Verification items for the finished model (mm, model axes). Face numbers are marked on the shaded views. Round coordinates to 2 decimals unless told otherwise and drop trailing zeros. Write each loop counter-clockwise with the first axis right and the second up, starting at its lowest first coordinate (ties: lowest second). Pieces come first, ordered by that corner, then holes. Notation, with made-up numbers: M -28.5,40 L 10.5,40 A25 cw 10.5,55 Z; hole C 0,83 d4. An arc over 180 degrees is marked long. Use a Markdown table: item, result. Add a question column.
Autodesk Inventor part; units mm, degrees
ref_plane "YZ Plane" through (0, 0, 0) normal (1, 0, 0) x (0, 1, 0)
ref_plane "XZ Plane" through (0, 0, 0) normal (0, 1, 0) x (-1, 0, 0)
ref_plane "XY Plane" through (0, 0, 0) normal (0, 0, 1) x (1, 0, 0)
sketch "Sketch1" plane through (0, 0, 0) normal (0, 0, 1) x (1, 0, 0)
  circle A0 centre (0, 0) radius 15
  circle A1 centre (0, 0) radius 55
  line L0 (15, 0) -> (55, 0) construction
  circle A2 centre (35, 0) radius 20 construction
  circle A3 centre (-17.5, 30.310889) radius 20 construction
  circle A4 centre (-17.5, -30.310889) radius 20 construction
  line L1 (0, 0) -> (-10.833994, 10.374226)
  line L2 (0, 0) -> (27.5, -47.631397)
  line L3 (0, 0) -> (-55, 0) construction
  line L4 (0, 0) -> (27.5, 47.631397)
  line L5 (17.5, 30.310889) -> (27.5, 47.631397) construction
  line L6 (-1.432373, 18.147489) -> (18.567627, 52.788505) construction
  line L7 (18.567627, 52.788505) -> (36.432373, 42.47429) construction
  line L8 (36.432373, 42.47429) -> (16.432373, 7.833273) construction
  line L9 (16.432373, 7.833273) -> (-1.432373, 18.147489) construction
  line L10 (-1.432373, 18.147489) -> (36.432373, 42.47429) construction
  line L11 (18.567627, 52.788505) -> (16.432373, 7.833273) construction
  line L12 (-1.48905, -18.180212) -> (18.51095, -52.821228) construction
  line L13 (18.51095, -52.821228) -> (36.48905, -42.441567) construction
  line L14 (36.48905, -42.441567) -> (16.48905, -7.80055) construction
  line L15 (16.48905, -7.80055) -> (-1.48905, -18.180212) construction
  line L16 (-1.48905, -18.180212) -> (36.48905, -42.441567) construction
  line L17 (18.51095, -52.821228) -> (16.48905, -7.80055) construction
  line L18 (-55.008072, 10.310889) -> (-15, 10.310889) construction
  line L19 (-15, 10.310889) -> (-15, -10.310889) construction
  line L20 (-15, -10.310889) -> (-55.008072, -10.310889) construction
  line L21 (-55.008072, -10.310889) -> (-55.008072, 10.310889)
  line L22 (-55.008072, 10.310889) -> (-15, -10.310889) construction
  line L23 (-15, 10.310889) -> (-55.008072, -10.310889) construction
  line L24 (-39.117828, -2.5) -> (-30.890244, -2.5) construction
  line L25 (-30.890244, -2.5) -> (-30.890244, 2.5) construction
  line L26 (-30.890244, 2.5) -> (-39.117828, 2.5) construction
  line L27 (-39.117828, 2.5) -> (-39.117828, -2.5) construction
  line L28 (-39.117828, -2.5) -> (-30.890244, 2.5) construction
  line L29 (-30.890244, -2.5) -> (-39.117828, 2.5) construction
  arc A5 (-10.89429, -10.310889) -> (-55.008072, -10.310889) centre (-32.951181, -37.548278) ccw
  line L30 (-55.008072, 10.310889) -> (-55.008072, -10.310889) construction
  arc A6 (-55.008072, 10.310889) -> (-10.833994, 10.374226) centre (-32.959623, 37.256893) ccw
  line L31 (-55.008072, 10.310889) -> (-55.008072, -10.310889) construction
  arc A7 (18.574544, -52.793832) -> (-3.567347, -14.569627) centre (-15.785604, -47.172317) ccw
  line L32 (36.433528, -42.482943) -> (18.574544, -52.793832)
  arc A8 (14.376637, -4.279288) -> (36.433528, -42.482943) centre (48.993353, -9.762421) ccw
  circle A9 centre (0, 0) radius 15
  arc A10 (36.433528, 42.482943) -> (14.401341, 4.195401) centre (48.745227, 9.915425) ccw
  line L33 (18.574544, 52.793832) -> (36.433528, 42.482943)
  arc A11 (-3.482347, 14.590177) -> (18.574544, 52.793832) centre (-16.042172, 47.310699) ccw
  circle A12 centre (0, 0) radius 15
  circle A13 centre (0, 0) radius 5
  point P0 (-27.5, 47.631397)
  point P1 (-27.5, -47.631397)
  point P2 (17.5, -30.310889)
  point P3 (-35.004036, 0)
  point P4 (-7.5, 12.990381)
  point P5 (-7.5, -12.990381)
  point P6 (-54.150171, 9.631146)
  point P7 (-54.1491, -9.637168)
  point P8 (-3.567347, -14.569627)
  point P9 (18.734269, -51.710997)
  point P10 (35.420582, -42.075912)
  point P11 (14.376637, -4.279288)
  point P12 (14.401341, 4.195401)
  point P13 (35.415903, 42.079851)
  point P14 (18.728517, 51.71308)
  point P15 (-3.482347, 14.590177)
  dimension "d0" = 30
  dimension "d1" = 40
  dimension "d4" = 360
  dimension "d6" = 5
  dimension "d9" = 360
  dimension "d11" = 10
sketch "Sketch1 outline for Extrusion1" plane through (0, 0, 0) normal (0, 0, 1) x (1, 0, 0)
  arc A0 (-10.833994, 10.374226) -> (-54.150171, 9.631146) centre (-32.959623, 37.256893) cw
  arc A1 (-3.482347, 14.590177) -> (-10.833994, 10.374226) centre (0, 0) ccw
  arc A2 (-54.150171, 9.631146) -> (-54.1491, -9.637168) centre (0, 0) ccw
  arc A3 (18.728517, 51.71308) -> (-3.482347, 14.590177) centre (-16.042172, 47.310699) cw
  arc A4 (-54.1491, -9.637168) -> (-10.89429, -10.310889) centre (-32.951181, -37.548278) cw
  arc A5 (35.415903, 42.079851) -> (18.728517, 51.71308) centre (0, 0) ccw
  arc A6 (-10.89429, -10.310889) -> (-3.567347, -14.569627) centre (0, 0) ccw
  arc A7 (14.401341, 4.195401) -> (35.415903, 42.079851) centre (48.745227, 9.915425) cw
  arc A8 (-3.567347, -14.569627) -> (18.734269, -51.710997) centre (-15.785604, -47.172317) cw
  arc A9 (14.376637, -4.279288) -> (14.401341, 4.195401) centre (0, 0) ccw
  arc A10 (18.734269, -51.710997) -> (35.420582, -42.075912) centre (0, 0) ccw
  arc A11 (35.420582, -42.075912) -> (14.376637, -4.279288) centre (48.993353, -9.762421) cw
  circle A12 centre (0, 0) radius 5
extrude "Extrusion1" add sketch "Sketch1 outline for Extrusion1" along normal blind 10
properties part number "Combine mk1"
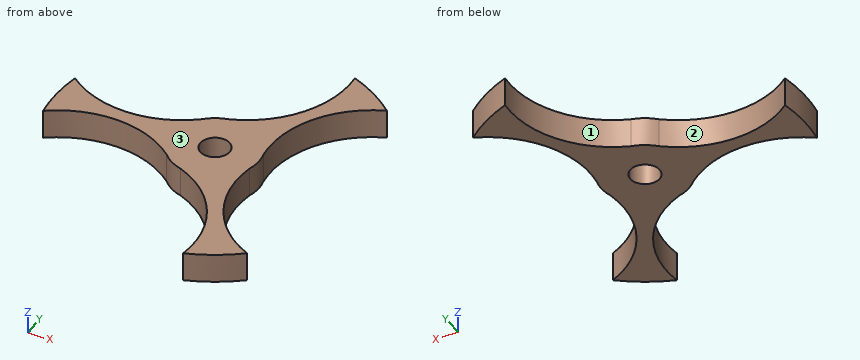
1. Cross-section at A-A on y = 0. Enter the section's corners in (x, z).
2. Depth check by flat-ended pin: pin 1 Ø5 at (x, z) = (-17, 3.5) entering from +Y; pin 2 Ø1 at (y, z) = (5, 8) entering from -X; pin 3 Ø2 at (y, z) = (-26.5, 1.5) entering from -X. Enter the tip coordinate at first touch or a pass-through.
3. Scan lines: line 1 along Y through (x, z) = (0, 3.25); line 2 along Y through (x, z) = (-0.5, 7.25); line 3 along X through (y, z) = (31, 2.25). Record each from-to range of solid material in increasing order. Write a range as from..to.
4. Cross-section at B-B on x = 0. Enter the section's corners in (y, z), plus the area to 3 significant figures.
5. Cross-section at D-D on x = 12.5. Enter the section's corners in (y, z), plus the area to 3 significant figures.
6. Release check for a two-part mould opening along X. For the marked faces 1, 2 and 3 record: +X half, -X half, draft (parallel to the pull), parting line (faces both ways), or undercut.
7. Cross-section at C-C on z = 5.25. Enter the section's corners in (x, y).
Answer:
| question | item | result |
|---|---|---|
| 1 | outline | M -55,0 L -5,0 L -5,10 L -55,10 Z; M 5,0 L 15,0 L 15,10 L 5,10 Z |
| 2 | pin 1 | stops at y = 7.74 |
| 2 | pin 2 | stops at x = -54.82 |
| 2 | pin 3 | stops at x = 11.46 |
| 3 | line 1 | y = -16.14..-5, 5..16.15 |
| 3 | line 2 | y = -15.89..-4.97, 4.97..15.9 |
| 3 | line 3 | x = 14.98..21.04 |
| 4 | outline | M -16.14,0 L -5,0 L -5,10 L -16.14,10 Z; M 5,0 L 16.15,0 L 16.15,10 L 5,10 Z |
| 4 | area | 223 mm^2 |
| 5 | outline | M -26.87,0 L 26.97,0 L 26.97,10 L -26.87,10 Z |
| 5 | area | 538 mm^2 |
| 6 | face 1 | -X half |
| 6 | face 2 | undercut |
| 6 | face 3 | draft |
| 7 | outline | M -54.15,-9.64 A35.05 cw -10.89,-10.31 A15 ccw -3.57,-14.57 A34.82 cw 18.73,-51.71 A55 ccw 35.42,-42.08 A35.05 cw 14.38,-4.28 A15 ccw 14.4,4.2 A34.82 cw 35.42,42.08 A55 ccw 18.73,51.71 A35.05 cw -3.48,14.59 A15 ccw -10.83,10.37 A34.82 cw -54.15,9.63 A55 ccw Z; hole C 0,0 d10 |
